```python
from build123d import *

# Parameters (mm, degrees)
BOSS_EXTRUDE1_DEPTH = 2
CUT_EXTRUDE1_DEPTH  = 2
SKETCH7_R           = 1.5
CUT_EXTRUDE3_DEPTH  = 2


with BuildPart() as part:
    # Sketch1 → Boss-Extrude1 (new body)
    with BuildSketch(Plane(origin=(0, 0, 0), x_dir=(1, 0, 0), z_dir=(0, 1, 0))):
        Polygon((0, 23.132168933), (-13.596747752, 18.714317784), (-22, 7.148233317), (-22, -7.148233317), (-13.596747752, -18.714317784), (0, -23.132168933), (13.596747752, -18.714317784), (22, -7.148233317), (22, 7.148233317), (13.596747752, 18.714317784), align=None)
    extrude(amount=BOSS_EXTRUDE1_DEPTH)

    # Sketch2 → Cut-Extrude1 (cut)
    with BuildSketch(Plane(origin=(0, 2, 0), x_dir=(1, 0, 0), z_dir=(0, 1, 0))):
        Polygon((0, 23.132168933), (-3.35, 22.043687951), (-3.35, 15.343687951), (3.35, 15.343687951), (3.35, 22.043687951), align=None)
        Polygon((11.729000424, 10.444223713), (15.667161615, 15.864637576), (13.596747752, 18.714317784), (10.246747752, 19.802798766), (6.308586562, 14.382384904), align=None)
        Polygon((15.627921341, 1.555421004), (22, 3.625834866), (22, 7.148233317), (19.929586138, 9.997913525), (13.557507479, 7.927499663), align=None)
        Polygon((13.557507479, -7.927499663), (19.929586138, -9.997913525), (22, -7.148233317), (22, -3.625834866), (15.627921341, -1.555421004), align=None)
        Polygon((6.308586562, -14.382384904), (10.246747752, -19.802798766), (13.596747752, -18.714317784), (15.667161615, -15.864637576), (11.729000424, -10.444223713), align=None)
        Polygon((-3.35, -15.343687951), (-3.35, -22.043687951), (0, -23.132168933), (3.35, -22.043687951), (3.35, -15.343687951), align=None)
        Polygon((-11.729000424, -10.444223713), (-15.667161615, -15.864637576), (-13.596747752, -18.714317784), (-10.246747752, -19.802798766), (-6.308586562, -14.382384904), align=None)
        Polygon((-15.627921341, -1.555421004), (-22, -3.625834866), (-22, -7.148233317), (-19.929586138, -9.997913525), (-13.557507479, -7.927499663), align=None)
        Polygon((-13.557507479, 7.927499663), (-19.929586138, 9.997913525), (-22, 7.148233317), (-22, 3.625834866), (-15.627921341, 1.555421004), align=None)
        Polygon((-6.308586562, 14.382384904), (-10.246747752, 19.802798766), (-13.596747752, 18.714317784), (-15.667161615, 15.864637576), (-11.729000424, 10.444223713), align=None)
    extrude(amount=-CUT_EXTRUDE1_DEPTH, mode=Mode.SUBTRACT)

    # Sketch7 → Cut-Extrude3 (cut)
    with BuildSketch(Plane(origin=(0, 2, 0), x_dir=(1, 0, 0), z_dir=(0, 1, 0))):
        with Locations(Location((0, 10, 0), (0, 0, 270))):
            Circle(SKETCH7_R)
        with Locations(Location((10, 0, 0), (0, 0, 270))):
            Circle(SKETCH7_R)
        with Locations(Location((0, -10, 0), (0, 0, 270))):
            Circle(SKETCH7_R)
        with Locations(Location((-10, 0, 0), (0, 0, 270))):
            Circle(SKETCH7_R)
    extrude(amount=-CUT_EXTRUDE3_DEPTH, mode=Mode.SUBTRACT)


solid = part.part
```
The listing builds one solid part. Answer for the finished solid, in the listing's coordinates (mm). A direction names the side the tool comes from. Coordinates: 2 decimals unless noted, no trailing zeros. Loops run counter-clockwise (first coordinate to the right, second up) from the corner with the lowest first, then second, coordinate; pieces in that order, holes last. Notation, with made-up numbers: (48, 32.5) -> (76, 32.5) arc R24 ccw to (76, 63.5) -> close; hole circle Ø3 at (74, 58.5). An arc over 180 degrees is marked (long way). Return JSON: item names as keys, results as strings. Group by question number.
(1) A cutting plane is placed at A-A on x = 0. Write down the section's boundary in (y, z).
(2) Find the intervals of material crossed by probe 1 along X at (y, z) = (1.25, 0); probe 2 along X at (y, z) = (1.3, -13); probe 3 along X at (y, z) = (1.15, -19.5), in increasing order. Write a range as from..to.
(3) Given pin 1 Ø1 at (y, z) = (1, 20) entering from -X; pin 2 Ø0.6 at (y, z) = (0.5, 19) entering from +X, each flat-ended and moving along its own axis, determine where each tip first touches the part or whether it passes through.
(4) A cutting plane is placed at D-D on z = 11. Write down the section's boundary in (x, y), and give its area (3 significant figures).
(5) A cutting plane is placed at B-B on z = 0. Write down the section's boundary in (x, y).
(6) Determine the mould class of faces 5 (the flat face through (6.847, 0.986, -20.908)), 6 (the flat face through (8.305, 1.014, -17.131)), 7 (the flat face through (-3.35, 1, 19)), 8 (the flat face through (0, 1, 15.344)) for opening direction Z: released by +Z, released by -Z, zero draft, split by the parting line, or undercut.
(7) Which of the six approach directions +Z, -Z, +X, -X, +Y, -Y give full straight-line access (tool end or side, diameter ignored) to faces 1 (the flat face through (0, 1, -15.344)), 2 (the flat face through (16.788, 1.014, -8.977)), 3 (the flat face through (-8.25, 1.014, -17.055)), 4 (the flat face through (0, 0, 0))?
(8) A cutting plane is placed at C-C on x = 9. Write down the section's boundary in (y, z).
The answers:
{
 "1": {"outline": "(0, -15.34) -> (2, -15.34) -> (2, -11.5) -> (0, -11.5) -> close; (0, -8.5) -> (2, -8.5) -> (2, 8.5) -> (0, 8.5) -> close; (0, 11.5) -> (2, 11.5) -> (2, 15.34) -> (0, 15.34) -> close"},
 "2": {"probe 1": "x = -22..-11.5, -8.5..8.5, 11.5..22", "probe 2": "x = -17.75..-13.59, -8.21..8.21, 13.59..17.75", "probe 3": "x = -10.03..-3.35, 3.35..10.03"},
 "3": {"pin 1": "stops at x = -10.25", "pin 2": "stops at x = 9.88"},
 "4": {"outline": "(-19.2, 0) -> (-12.13, 0) -> (-12.13, 2) -> (-19.2, 2) -> close; (-10.96, 0) -> (-1.12, 0) -> (-1.12, 2) -> (-10.96, 2) -> close; (1.12, 0) -> (10.96, 0) -> (10.96, 2) -> (1.12, 2) -> close; (12.13, 0) -> (19.2, 0) -> (19.2, 2) -> (12.13, 2) -> close", "area": "67.7 mm^2"},
 "5": {"outline": "(-22, 0) -> (-11.5, 0) -> (-11.5, 2) -> (-22, 2) -> close; (-8.5, 0) -> (8.5, 0) -> (8.5, 2) -> (-8.5, 2) -> close; (11.5, 0) -> (22, 0) -> (22, 2) -> (11.5, 2) -> close"},
 "6": {"face 5": "released by -Z", "face 6": "undercut", "face 7": "zero draft", "face 8": "released by +Z"},
 "7": {"face 1": "-Z, +Y, -Y", "face 2": "+X, +Y, -Y", "face 3": "+Y, -Y", "face 4": "+Z, -Z, +X, -X, -Y"},
 "8": {"outline": "(0, -20.21) -> (2, -20.21) -> (2, -18.09) -> (0, -18.09) -> close; (0, -12.43) -> (2, -12.43) -> (2, -1.12) -> (0, -1.12) -> close; (0, 1.12) -> (2, 1.12) -> (2, 12.43) -> (0, 12.43) -> close; (0, 18.09) -> (2, 18.09) -> (2, 20.21) -> (0, 20.21) -> close"}
}
